The drawing under review shows one solid part. Ordinate dimensions are in mm from its lowest x, y, z. A direction names the side the tool comes from. Coordinates: 2 decimals unless noted, no trailing zeros. Order: outer loops, then holes, each group sorted by start corner. A loop starts at its lowest first (then second) coordinate and runs counter-clockwise, first axis right, second up.
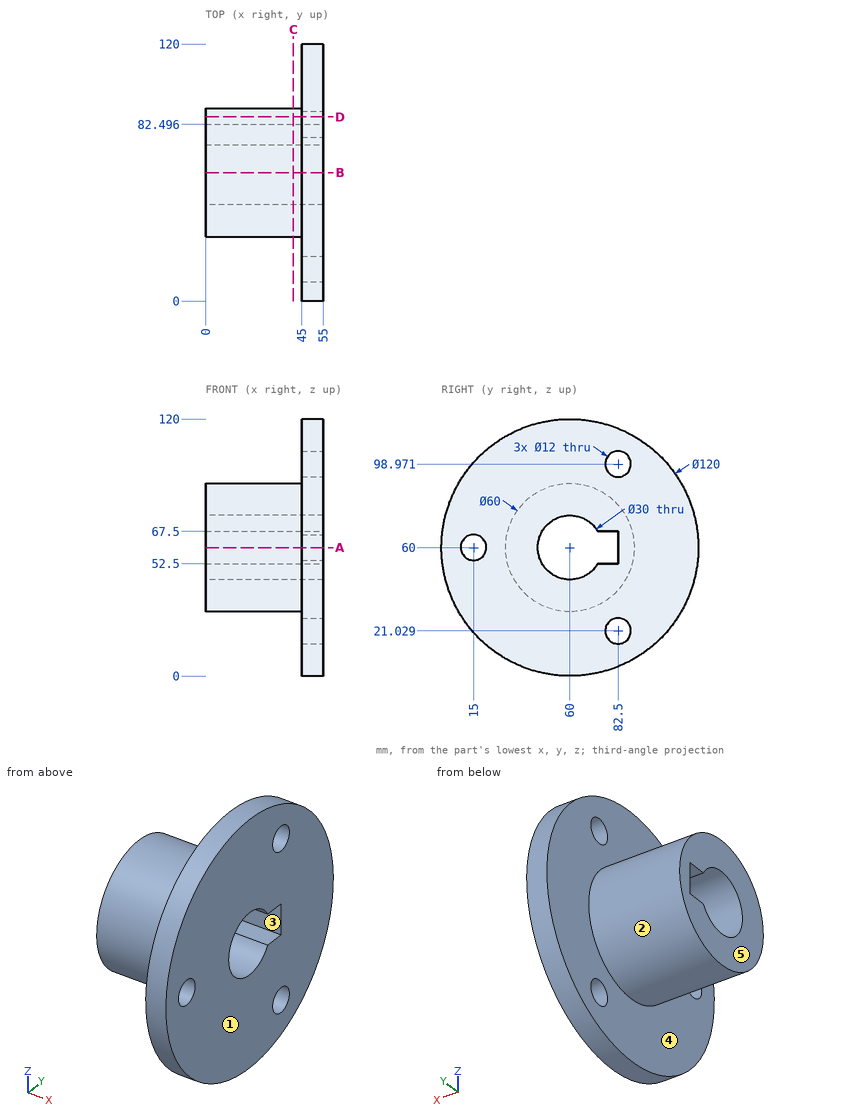
(1) Wall thickness on probe 1 along Y at (x, z) = (49.5, 60) (1 decimal); probe 2 along X at (y, z) = (73, 14); probe 3 along Z at (x, y) = (36, 77): over which ranges is each line inside the solid? List them lowest first.
A:
probe 1: y = 0 to 9, 21 to 45, 82.5 to 120
probe 2: x = 45 to 55
probe 3: z = 35.28 to 52.5, 67.5 to 84.72
(2) Draft analysis for pull direction Y (two halves, no side actions). For the marked faces 1, 2 and 3, state which applies: released by +Y, released by -Y, zero draft, split by the parting line, or undercut.
A:
face 1: zero draft
face 2: split by the parting line
face 3: undercut
(3) We need section D-D, the plane y = 86. Write out the cut boundary in (x, z) (1 decimal), and give its area (3 significant figures).
A:
outline: (0, 45) - (45, 45) - (45, 25.9) - (55, 25.9) - (55, 94.1) - (45, 94.1) - (45, 75) - (0, 75) - close; (45, 5.9) - (55, 5.9) - (55, 16.2) - (45, 16.2) - close; (45, 103.8) - (55, 103.8) - (55, 114.1) - (45, 114.1) - close
area: 2,230 mm2
(4) For pin 1 Ø11 at (y, z) = (15, 60) entering from +X; pin 2 Ø10.5 at (x, y) = (24, 77) entering from +Z; pin 3 Ø7.5 at (x, y) = (36.5, 78) entering from -Z; pin 4 Ø3 at (x, z) = (45.5, 93.5) entering from -Y (1 decimal), all flat-tipped, find the tip position at first contact; note any pin that passes through.
A:
pin 1: passes through
pin 2: stops at z = 87.6
pin 3: stops at z = 33.6
pin 4: stops at y = 9.2
(5) We need section B-B, the plane y = 60. Write out the cut boundary in (x, z).
A:
outline: (0, 30) - (45, 30) - (45, 0) - (55, 0) - (55, 45) - (0, 45) - close; (0, 75) - (55, 75) - (55, 120) - (45, 120) - (45, 90) - (0, 90) - close
(6) We need section A-A, the plane z = 60. Write out the cut boundary in (x, y) (1 decimal).
A:
outline: (0, 30) - (45, 30) - (45, 21) - (55, 21) - (55, 45) - (0, 45) - close; (0, 82.5) - (55, 82.5) - (55, 120) - (45, 120) - (45, 90) - (0, 90) - close; (45, 0) - (55, 0) - (55, 9) - (45, 9) - close
(7) Machinability: for the marked faces 4 and 5, which of the approach directions +Z, -Z, +X, -X, +Y, -Y give a long, thin tool a straight path to every point of the face, cutting with its end or side? Answer none if there is none.
A:
face 4: -X
face 5: +Z, -Z, -X, +Y, -Y
(8) We need section C-C, the plane x = 41. Write out the cut boundary in (y, z) (1 decimal), and give its area (3 significant figures).
A:
outline: circle Ø60 at (60, 60); hole (73, 52.5) - (82.5, 52.5) - (82.5, 67.5) - (73, 67.5) arc R15 ccw (long way) to start
area: 2,000 mm2
